Study the drawing (mm; zero at the part's minimum x, y, z) and answer. A direction names the side the tool comes from. Round coordinates to 2 decimals unless told otherwise and drop trailing zeros. Loops run counter-clockwise (first coordinate to the right, second up) from the corner with the lowest first, then second, coordinate; pieces in that order, holes last. Notation, with made-up numbers: (64.25, 75) - (100.25, 75) arc R10 cw to (100.25, 83) - close; hole circle Ø9 at (-9.5, 24.25). An arc over 180 degrees is marked (long way). One line per item, written item: value.
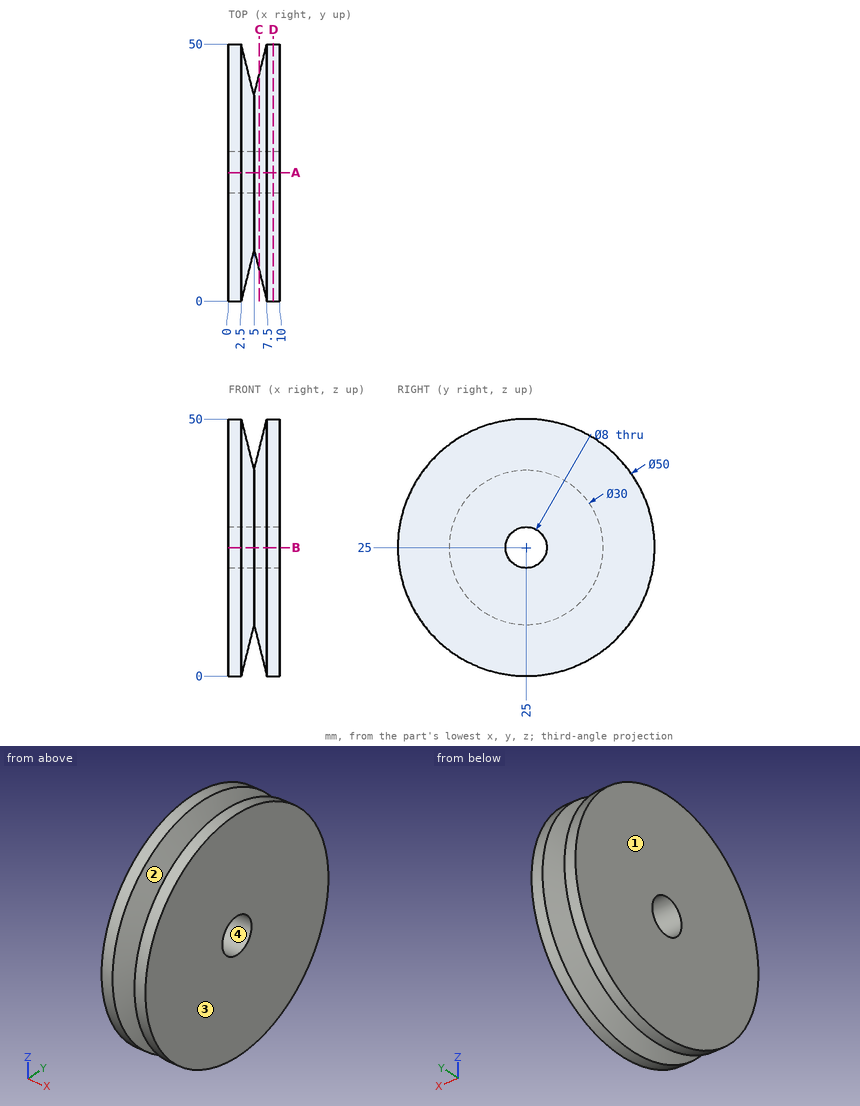
1) A cutting plane is placed at C-C on x = 6. Give the vertices of the cut face in (y, z).
Final values:
outline: circle Ø38 at (25, 25); hole circle Ø8 at (25, 25)
2) Each of these flat-tipped pins is pushed along its axis until it touches: pin 1 Ø5 at (x, y) = (3.5, 42.5) entering from -Z; pin 2 Ø6 at (x, z) = (6, 42) entering from -Y; pin 3 Ø2 at (x, y) = (2, 37.5) entering from +Z. Where does it stop, or does it pass through?
Final values:
pin 1: z = 5.16
pin 2: y = 4.57
pin 3: z = 47.2
3) For a pull along Z with two mould halves and no side action, classify the marked faces 3 and 4 as released by +Z, released by -Z, zero draft, split by the parting line, or undercut.
Final values:
face 3: zero draft
face 4: undercut
4) A cutting plane is placed at A-A on y = 25. Give the vertices of the cut face in (x, z).
Final values:
outline: (0, 0) - (2.5, 0) - (5, 10) - (7.5, 0) - (10, 0) - (10, 21) - (0, 21) - close; (0, 29) - (10, 29) - (10, 50) - (7.5, 50) - (5, 40) - (2.5, 50) - (0, 50) - close
5) A cutting plane is placed at D-D on x = 8.75. Give the vertices of the cut face in (y, z), and give its area (3 significant figures).
Final values:
outline: circle Ø50 at (25, 25); hole circle Ø8 at (25, 25)
area: 1,910 mm2
6) Consider L1, parallel to X at y = 42, z = 34.5; L2, parallel to X at y = 37, z = 34.5; L3, parallel to Z at x = 1.25, y = 34. Determine where each line is inside the solid, lowest interval first.
Final values:
L1: 0 to 3.88, 6.12 to 10
L2: 0 to 4.92, 5.08 to 10
L3: 1.68 to 48.32
7) For the marked faces 1 and 2, determine the directions among +Z, -Z, +X, -X, +Y, -Y from which every point of the face is accessible in a straight line to the end or side of a thin tool.
Final values:
face 1: +Z, -Z, -X, +Y, -Y
face 2: none
